from build123d import *

# Parameters (mm, degrees)
F1_DEPTH = 12.7
F3_D     = 3.81


with BuildPart() as f1:
    # F0 (on Front) → F1 (new body, symmetric)
    with BuildSketch(Plane.XZ):
        Polygon((0, 27.94), (0, 0), (-3.81, 0), (-3.81, 3.81), (-6.35, 3.81), (-6.35, -5.334), (19.05, -12.139909), (19.05, 38.660091), (-6.35, 31.854181), (-6.35, 24.13), (-3.81, 24.13), (-3.81, 27.94), align=None)
    extrude(amount=F1_DEPTH, both=True)

    # F3 (through all)
    with Locations(Plane(origin=(0, 0, 0), x_dir=(0, -1, 0), z_dir=(-1, 0, 0))):
        with Locations((0, 13.260091)):
            Hole(F3_D / 2)


solid = f1.part
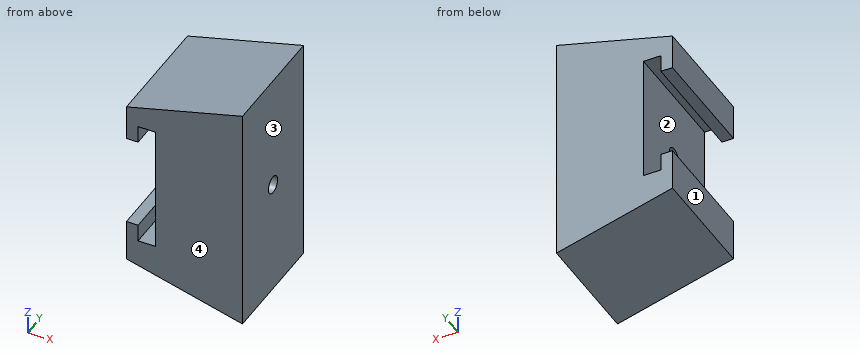
Geometry check sheet. Reference: the model listing, model coordinates, mm. Face numbers are marked on the shaded views. Round coordinates to 2 decimals unless told otherwise and drop trailing zeros. Order: outer loops, then holes, each group sorted by start corner. A loop starts at its lowest first (then second) coordinate and runs counter-clockwise, first axis right, second up. Notation, with made-up numbers: (49, 87) - (80, 87) arc R13 ccw to (80, 101) - close; hole circle Ø9 at (-22.5, -4.5). An arc over 180 degrees is marked (long way). One line per question, with ' | ' between items. Start each with the question number.
(1) Sectioned sample at B-B on z = 2. Record the cut outline in (x, y), and give its area (3 significant figures).
(2) Depth check by flat-ended pin: pin 1 Ø0.8 at (x, y) = (-5, 2) entering from +Z; pin 2 Ø8 at (x, y) = (14.5, 4) entering from +Z; pin 3 Ø1.9 at (x, y) = (-1.5, -5.5) entering from +Z. Enter the tip coordinate at first touch or a pass-through.
(3) Sectioned sample at D-D on y = -6. Record the cut outline in (x, z).
(4) Sectioned sample at A-A on y = 0. Record the cut outline in (x, z), and give its area (3 significant figures).
(5) Sectioned sample at C-C on x = -1.25. Record the cut outline in (y, z), and give its area (3 significant figures).
(6) Release check for a two-part mould opening along X. For the marked faces 1, 2, 3 and 4 record: released by +X, released by -X, zero draft, split by the parting line, or undercut.
(7) Thickness scan on L1, parallel to X at y = 8.5, z = 2.5; L2, parallel to X at y = 7.25, z = 14.5; L3, parallel to Z at x = 4, y = 0. Record the ranges inside material, lowest first. Write a range as [from, to].
Conclusion:
1) outline: (-6.35, -12.7) - (-3.81, -12.7) - (-3.81, 12.7) - (-6.35, 12.7) - close; (0, -12.7) - (19.05, -12.7) - (19.05, 12.7) - (0, 12.7) - close | area: 548 mm2
2) pin 1: stops at z = 32.32 | pin 2: stops at z = 38.51 | pin 3: stops at z = 33.41
3) outline: (-6.35, -5.33) - (19.05, -12.14) - (19.05, 38.66) - (-6.35, 31.85) - (-6.35, 24.13) - (-3.81, 24.13) - (-3.81, 27.94) - (0, 27.94) - (0, 0) - (-3.81, 0) - (-3.81, 3.81) - (-6.35, 3.81) - close
4) outline: (-6.35, -5.33) - (19.05, -12.14) - (19.05, 11.36) - (0, 11.36) - (0, 0) - (-3.81, 0) - (-3.81, 3.81) - (-6.35, 3.81) - close; (-6.35, 24.13) - (-3.81, 24.13) - (-3.81, 27.94) - (0, 27.94) - (0, 15.17) - (19.05, 15.17) - (19.05, 38.66) - (-6.35, 31.85) - close | area: 887 mm2
5) outline: (-12.7, -6.7) - (12.7, -6.7) - (12.7, 0) - (-12.7, 0) - close; (-12.7, 27.94) - (12.7, 27.94) - (12.7, 33.22) - (-12.7, 33.22) - close | area: 304 mm2
6) face 1: released by -X | face 2: undercut | face 3: released by +X | face 4: zero draft
7) L1: x = [-6.35, -3.81], [0, 19.05] | L2: x = [0, 19.05] | L3: z = [-8.11, 11.36], [15.17, 34.63]
